```python
from build123d import *

# Parameters (mm, degrees)
ESQUISSE1_W        = 118
ESQUISSE1_H        = 18
ESQUISSE1_R        = 3.5
BOSS_EXTRU_1_DEPTH = 6
CONG_1_R           = 9


with BuildPart() as part:
    # Esquisse1 → Boss.-Extru.1 (new body)
    with BuildSketch(Plane.XY):
        with Locations((59, 9)):
            Rectangle(ESQUISSE1_W, ESQUISSE1_H)
        with Locations((9, 9)):
            Circle(ESQUISSE1_R, mode=Mode.SUBTRACT)
        with Locations(Location((109, 9, 0), (0, 0, 180))):
            Circle(ESQUISSE1_R, mode=Mode.SUBTRACT)
    extrude(amount=BOSS_EXTRU_1_DEPTH)

    # Congé1
    cong_1_edges = [part.edges().sort_by_distance(p)[0] for p in [
        (118, 18, 3),
        (118, 0, 3),
        (0, 0, 3),
        (0, 18, 3),
    ]]
    fillet(cong_1_edges, radius=CONG_1_R - 0.0001)  # a hair under: the kernel refuses the full size


solid = part.part
```
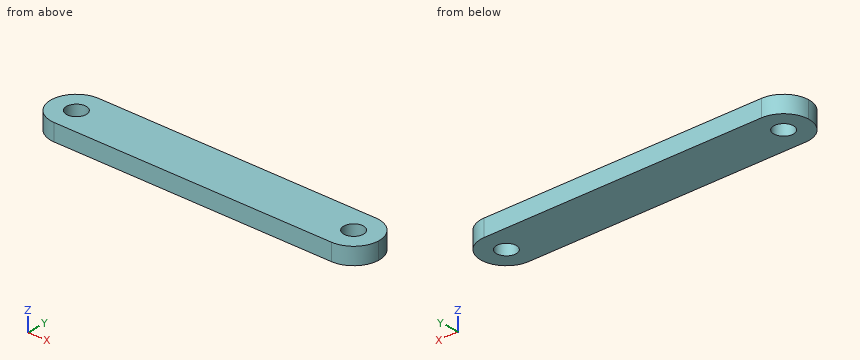
Work out the finished part from the listing and answer in its coordinate system (mm). Round coordinates to 2 decimals unless told otherwise and drop trailing zeros. Loops run counter-clockwise (first coordinate to the right, second up) from the corner with the lowest first, then second, coordinate; pieces in that order, holes last.
(1) The part is cut by section B-B, the plane y = 2. Give the vertices of the cut face in (x, z).
Computed values:
outline: (3.34, 0) - (114.66, 0) - (114.66, 6) - (3.34, 6) - close
(2) The part is cut by section A-A, the plane y = 8. Give the vertices of the cut face in (x, z).
Computed values:
outline: (0.06, 0) - (5.65, 0) - (5.65, 6) - (0.06, 6) - close; (12.35, 0) - (105.65, 0) - (105.65, 6) - (12.35, 6) - close; (112.35, 0) - (117.94, 0) - (117.94, 6) - (112.35, 6) - close
(3) Each of these flat-tipped pins is pushed along its axis until it touches: P1, Ø1, axis at y = 12.5, z = 3, coming from the -X side; P2, Ø1.5, axis at y = 2, z = 4.5, coming from the +X side; P3, Ø4, axis at x = 35, y = 3.5, coming from the -Z side. Where does it stop, or does it pass through?
Computed values:
P1: stops at x = 0.51
P2: stops at x = 115.48
P3: stops at z = 0
(4) Find the intervals of material crossed by L1, parallel to Y at x = 9, z = 4.3; L2, parallel to X at y = 11, z = 5.6; L3, parallel to X at y = 6.75, z = 0.35, in increasing order.
Computed values:
L1: y = 0 to 5.5, 12.5 to 18
L2: x = 0.23 to 6.13, 11.87 to 106.13, 111.87 to 117.77
L3: x = 0.29 to 6.32, 11.68 to 106.32, 111.68 to 117.71
